The figure shows three views and two pictorial views of one solid part (mm, origin at its lowest corner). Answer the questions. Give positions to 0.01 mm unless a question says otherwise; leave off trailing zeros. Write each loop counter-clockwise with the first axis right and the second up, starting at its lowest first coordinate (ties: lowest second). Pieces come first, ordered by that corner, then holes. Notation, with made-up numbers: M 15.25,47.25 L 66.25,47.25 A23 ccw 66.25,74.25 Z; hole C 73.25,-9.75 d10. An arc over 180 degrees is marked long. Return JSON: item names as keys, results as strings.
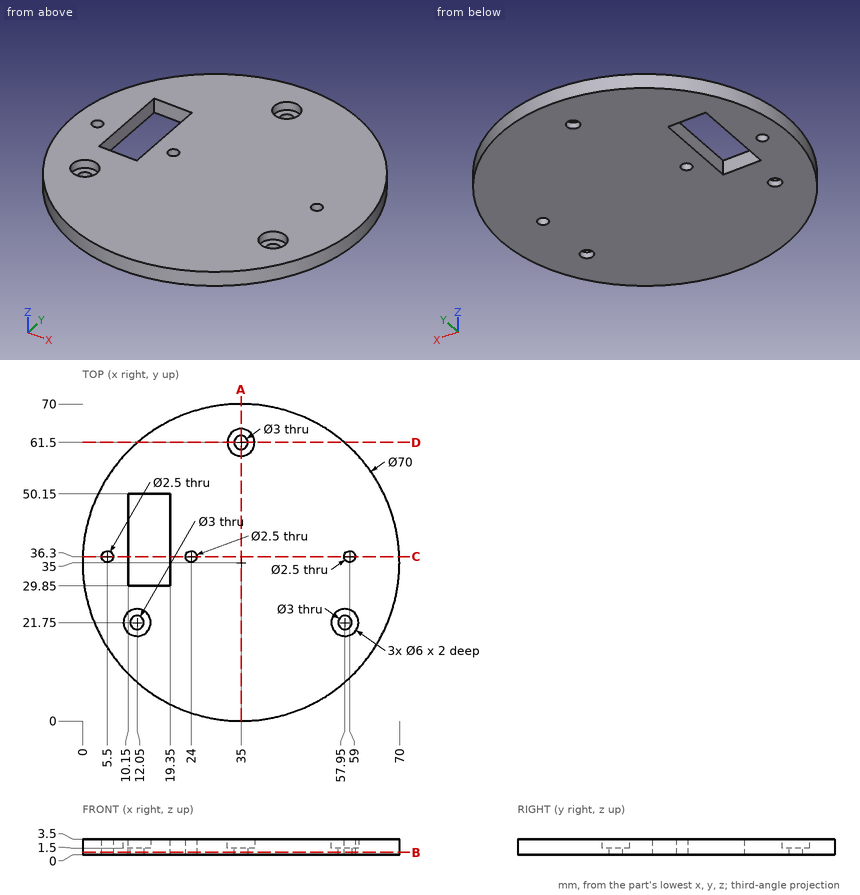
Item 1: A cutting plane is placed at C-C, the plane y = 36.3. Write down the section's boundary in (x, z).
Geometry results:
{"outline": "M 0.02,0 L 4.25,0 L 4.25,3.5 L 0.02,3.5 Z; M 6.75,0 L 10.15,0 L 10.15,3.5 L 6.75,3.5 Z; M 19.35,0 L 22.75,0 L 22.75,3.5 L 19.35,3.5 Z; M 25.25,0 L 57.75,0 L 57.75,3.5 L 25.25,3.5 Z; M 60.25,0 L 69.98,0 L 69.98,3.5 L 60.25,3.5 Z"}
Item 2: A cutting plane is placed at D-D, the plane y = 61.5. Write down the section's boundary in (x, z).
Geometry results:
{"outline": "M 12.14,0 L 33.5,0 L 33.5,1.5 L 32,1.5 L 32,3.5 L 12.14,3.5 Z; M 36.5,0 L 57.86,0 L 57.86,3.5 L 38,3.5 L 38,1.5 L 36.5,1.5 Z"}
Item 3: A cutting plane is placed at B-B, the plane z = 0.55. Write down the section's boundary in (x, y).
Geometry results:
{"outline": "C 35,35 d70; hole C 5.5,36.3 d2.5; hole M 10.15,29.85 L 19.35,29.85 L 19.35,50.15 L 10.15,50.15 Z; hole C 12.05,21.75 d3; hole C 24,36.3 d2.5; hole C 35,61.5 d3; hole C 57.95,21.75 d3; hole C 59,36.3 d2.5"}
Item 4: Find the intervals of material crossed by line 1 (X direction, y = 34, z = 1.9); line 2 (Y direction, x = 35, z = 0.7); line 3 (Y direction, x = 13, z = 0.2), in increasing order.
Geometry results:
{"line 1": "x = 0.01 to 10.15, 19.35 to 69.99", "line 2": "y = 0 to 60, 63 to 70", "line 3": "y = 7.78 to 20.59, 22.91 to 29.85, 50.15 to 62.22"}
Item 5: A cutting plane is placed at A-A, the plane x = 35. Write down the section's boundary in (y, z).
Geometry results:
{"outline": "M 0,0 L 60,0 L 60,1.5 L 58.5,1.5 L 58.5,3.5 L 0,3.5 Z; M 63,0 L 70,0 L 70,3.5 L 64.5,3.5 L 64.5,1.5 L 63,1.5 Z"}
Item 6: Given pin 1 Ø5 at (x, y) = (12.5, 22.5) entering from +Z; pin 2 Ø1 at (x, z) = (55, 0.5) entering from -Y (1 decimal); pin 3 Ø2 at (y, z) = (31, 2) entering from -X, each flat-ended and moving along its own axis, determine where each tip first touches the part or whether it passes through.
Geometry results:
{"pin 1": "stops at z = 3.5", "pin 2": "stops at y = 5.9", "pin 3": "stops at x = 0.13"}
